Read the model definition and answer for the solid it produces. Units are mm, in the model's axes. A direction names the side the tool comes from. Give positions to 0.01 mm unless a question says otherwise; leave off trailing zeros. Order: outer loops, then holes, each group sorted by start corner. A loop starts at its lowest first (then second) coordinate and runs counter-clockwise, first axis right, second up. Notation, with made-up numbers: (70, 45) - (90, 45) arc R19 ccw to (90, 51) - close; hole circle Ø7 at (18, 55.5). An arc over 180 degrees is marked (long way). Write each question's results on one line, items separated by ' | '.
from build123d import *

# Parameters (mm, degrees)
RESSALTO_EXTRUS_O1_DEPTH      = 26
RESSALTO_EXTRUS_O1_DEPTH_BACK = 26
ESBO_O10_R                    = 6
ESBO_O10_R_2                  = 3
CASCA1_START                  = -21.5
CASCA1_OUTLINE_R              = 10.5
CASCA1_DEPTH                  = 43
CORTE_EXTRUS_O1_DEPTH         = 111.580287574
CORTE_EXTRUS_O1_DEPTH_BACK    = 111.580287574
ESBO_O12_W                    = 43
ESBO_O12_H                    = 35.359478928
FILETE3_R                     = 9
ESBO_O17_W                    = 71.509931374
ESBO_O17_H                    = 43
CORTE_EXTRUS_O6_DEPTH         = 20
FILETE7_R                     = 3
FILETE8_R                     = 3
FILETE9_R                     = 12
ESBO_O18_W                    = 3
ESBO_O18_H                    = 14
CORTE_EXTRUS_O7_DEPTH         = 10
CORTE_EXTRUS_O8_DEPTH         = 120.398492453
CORTE_EXTRUS_O8_DEPTH_BACK    = 120.398492453
ESBO_O19_R                    = 3
FILETE10_R                    = 10
ESBO_O20_R                    = 2
CORTE_EXTRUS_O10_DEPTH        = 10


# Read off the part's stored shape, not the designer's step: Casca1
with BuildPart() as part:
    # Esboço10 → Ressalto-extrusão1 (new, two sides: drawn at the far end of the back side and taken through both)
    with BuildSketch(Plane.XY.offset(-RESSALTO_EXTRUS_O1_DEPTH_BACK)):
        with BuildLine():
            Line((8.831023296, -7.34936003), (73.857380106, 62.551046129))
            ThreePointArc((73.857380106, 62.551046129), (75.334563074, 71.194398928), (68, 76))
            Line((68, 76), (25.460219944, 76))
            Line((25.460219944, 76), (25.460219944, 69))
            Line((25.460219944, 69), (3.255321751, 69))
            Line((3.255321751, 69), (3.255321751, 76))
            Line((3.255321751, 76), (-46.744678249, 76))
            Line((-46.744678249, 76), (-10.47981176, -4.708886362))
            ThreePointArc((-10.47981176, -4.708886362), (-1.556486796, -11.383207552), (8.831023296, -7.34936003))
        make_face()
        Circle(ESBO_O10_R, mode=Mode.SUBTRACT)
        with Locations((68, 68)):
            Circle(ESBO_O10_R_2, mode=Mode.SUBTRACT)
    extrude(amount=RESSALTO_EXTRUS_O1_DEPTH + RESSALTO_EXTRUS_O1_DEPTH_BACK)

    # Casca1 outline → Casca1 (cut)
    with BuildSketch(Plane.XY.offset(CASCA1_START)):
        with BuildLine():
            Line((8.831023296, -7.34936003), (73.857380106, 62.551046129))
            Line((73.857380106, 62.551046129), (73.491293849, 62.891605746))
            ThreePointArc((73.491293849, 62.891605746), (63.658096197, 61.884620096), (61.366750419, 71.5))
            Line((61.366750419, 71.5), (29.960219944, 71.5))
            Line((29.960219944, 71.5), (29.960219944, 64.5))
            Line((29.960219944, 64.5), (-1.244678249, 64.5))
            Line((-1.244678249, 64.5), (-1.244678249, 71.5))
            Line((-1.244678249, 71.5), (-44.722696451, 71.5))
            Line((-44.722696451, 71.5), (-10.47981176, -4.708886362))
            ThreePointArc((-10.47981176, -4.708886362), (-1.556486796, -11.383207552), (8.831023296, -7.34936003))
        make_face()
        Circle(CASCA1_OUTLINE_R, mode=Mode.SUBTRACT)
    extrude(amount=CASCA1_DEPTH, mode=Mode.SUBTRACT)

    # Esboço12 → Corte-extrusão1 (cut, two sides: drawn at the far end of the back side and taken through both)
    with BuildSketch(Plane(origin=(0, 0, 0), x_dir=(0, 0, -1), z_dir=(1, 0, 0)).offset(-CORTE_EXTRUS_O1_DEPTH_BACK)):
        Rectangle(ESBO_O12_W, ESBO_O12_H)
    extrude(amount=CORTE_EXTRUS_O1_DEPTH + CORTE_EXTRUS_O1_DEPTH_BACK, mode=Mode.SUBTRACT)

    # Filete3
    # the kernel refuses this fillet: 9 mm, written as the material it takes off along each edge
    with BuildSketch(Plane(origin=(-1.244678249, 64.5, -21.5), x_dir=(0, 1, 0), z_dir=(0, 0, 1))) as filete3_piece_1:
        with BuildLine():
            CenterArc((9, -8.774964387), FILETE3_R, 102.839588407, 77.160411593)
            Line((0, -8.774964387), (0, 0))
            Line((0, 0), (7, 0))
        make_face()
    extrude(amount=43, mode=Mode.SUBTRACT)

    # Esboço17 → Corte-extrusão6 (cut)
    with BuildSketch(Plane(origin=(0, 76, 0), x_dir=(1, 0, 0), z_dir=(0, 1, 0))):
        with Locations((61.215185631, 0)):
            Rectangle(ESBO_O17_W, ESBO_O17_H)
    extrude(amount=-CORTE_EXTRUS_O6_DEPTH, mode=Mode.SUBTRACT)

    # Filete7
    filete7_edges = [part.edges().sort_by_distance(p)[0] for p in [
        (25.460219944, 76, 23.75),
        (25.460219944, 76, -23.75),
    ]]
    fillet(filete7_edges, radius=FILETE7_R)

    # Filete8
    filete8_edges = [part.edges().sort_by_distance(p)[0] for p in [
        (3.255321751, 76, 0),
    ]]
    fillet(filete8_edges, radius=FILETE8_R)

    # Filete9
    # the kernel refuses this fillet: 12 mm, written as the material it takes off along each edge
    with BuildSketch(Plane(origin=(25.460219944, 69, -21.5), x_dir=(-1, 0, 0), z_dir=(0, 0, 1))) as filete9_piece_1:
        with BuildLine():
            CenterArc((9.367496998, 12), FILETE9_R, 218.682187453, 51.317812547)
            Line((0, 4.5), (0, 0))
            Line((0, 0), (9.367496998, 0))
        make_face()
    extrude(amount=43, mode=Mode.SUBTRACT)

    # Esboço18 → Corte-extrusão7 (cut)
    with BuildSketch(Plane(origin=(0, 69, 0), x_dir=(1, 0, 0), z_dir=(0, 1, 0))):
        with Locations((14.592722946, 0)):
            Rectangle(ESBO_O18_W, ESBO_O18_H)
    extrude(amount=-CORTE_EXTRUS_O7_DEPTH, mode=Mode.SUBTRACT)

    # Esboço19 → Corte-extrusão8 (cut, two sides: drawn at the far end of the back side and taken through both)
    with BuildSketch(Plane.XY.offset(26).offset(-CORTE_EXTRUS_O8_DEPTH_BACK)):
        with Locations((-33.678552977, 64)):
            Circle(ESBO_O19_R)
    extrude(amount=CORTE_EXTRUS_O8_DEPTH + CORTE_EXTRUS_O8_DEPTH_BACK, mode=Mode.SUBTRACT)

    # Filete10
    filete10_edges = [part.edges().sort_by_distance(p)[0] for p in [
        (25.460219944, 69, -23.75),
        (25.460219944, 69, 23.75),
    ]]
    fillet(filete10_edges, radius=FILETE10_R)

    # Esboço20 → Corte-extrusão10 (cut)
    with BuildSketch(Plane(origin=(0, 76, 0), x_dir=(1, 0, 0), z_dir=(0, 1, 0))):
        with Locations(Location((-27.244678249, 14.25, 0), (0, 0, 180))):
            Circle(ESBO_O20_R)
        with Locations(Location((-27.244678249, -14.25, 0), (0, 0, 180))):
            Circle(ESBO_O20_R)
    extrude(amount=-CORTE_EXTRUS_O10_DEPTH, mode=Mode.SUBTRACT)


solid = part.part
(1) For faces 5 (the face through (-23, 71.5, 0)), 6 (the face through (3.255, 71, 0)), 7 (the face through (15, 67, -7)), 8 (the face through (21.36, 67.78, -0.3)), determine the directions among +Z, -Z, +X, -X, +Y, -Y from which every point of the face is accessible in a straight line to the end or side of a thin tool.
Conclusion:
face 5: -X, -Y | face 6: +Z, -Z, +Y | face 7: +Y, -Y | face 8: +X, +Y
(2) Consider probe 1 along Z at (x, y) = (-14, 46); probe 2 along Y at (x, z) = (-17, 9); probe 3 along X at (y, z) = (64, -24.2). Determine where each line is inside the solid, lowest interval first. Write a range as [from, to].
Conclusion:
probe 1: [-26, -21.5], [21.5, 26] | probe 2: [71.5, 76] | probe 3: [-41.35, -36.68], [-30.68, 74.93]
(3) Section A-A (z = 14.25) is taken. Give the vertices of the cut face in (x, y), plus the area to 3 significant figures.
Conclusion:
outline: (-46.74, 76) - (-44.72, 71.5) - (-29.24, 71.5) - (-29.24, 76) - close; (-25.24, 71.5) - (-1.24, 71.5) arc R9 ccw to (7.53, 64.5) - (25.46, 64.5) arc R12 ccw to (16.09, 69) - (3.26, 69) - (3.26, 73) arc R3 ccw to (0.26, 76) - (-25.24, 76) - close | area: 303 mm^2
(4) Section D-D (y = 8.5) is taken. Give the vertices of the cut face in (x, z).
Conclusion:
outline: (-16.41, -26) - (23.58, -26) - (23.58, -21.5) - (-16.41, -21.5) - close; (-16.41, 21.5) - (23.58, 21.5) - (23.58, 26) - (-16.41, 26) - close
(5) Section B-B (y = -1.5) is taken. Give the vertices of the cut face in (x, z).
Conclusion:
outline: (-11.92, -26) - (-5.81, -26) - (-5.81, -21.5) - (-11.92, -21.5) - close; (-11.92, 21.5) - (-5.81, 21.5) - (-5.81, 26) - (-11.92, 26) - close; (5.81, -26) - (14.27, -26) - (14.27, -21.5) - (5.81, -21.5) - close; (5.81, 21.5) - (14.27, 21.5) - (14.27, 26) - (5.81, 26) - close
(6) The mould has two halves that part along Y. Classify faces 1 (the face through (-23, 76, 0)), 2 (the face through (65.6, 66.2, -23.8)), 3 (the face through (-32.726, 44.802, 22.99)), 4 (the face through (15, 67, 7)): pulls with the +Y half, pulls with the -Y half, needs draft (parallel to the pull), parting line crosses it, or undercut.
Conclusion:
face 1: pulls with the +Y half | face 2: undercut | face 3: pulls with the -Y half | face 4: needs draft
(7) Section C-C (x = 54) is taken. Give the vertices of the cut face in (y, z), plus the area to 3 significant figures.
Conclusion:
outline: (41.21, -26) - (76, -26) - (76, -21.5) - (41.21, -21.5) - close; (41.21, 21.5) - (76, 21.5) - (76, 26) - (41.21, 26) - close | area: 313 mm^2
(8) Each of these flat-tipped pins is pushed along its axis until it touches: pin 1 (4 mm diameter, centred on x = 13, z = 5.5, fed in from +Y); pin 2 (5 mm diameter, centred on y = 66.5, z = -1, fed in from +X); pin 3 (6 mm diameter, centred on x = -25, z = 11.5, fed in from -Y). Where does it stop, or does it pass through?
Conclusion:
pin 1: y = 69 | pin 2: x = 25.46 | pin 3: y = 71.5
